Can you work these out from the model? Positions are in its coordinate system, mm. Face numbers are marked on the shaded views. Coordinates: 2 decimals unless noted, no trailing zeros. Loops run counter-clockwise (first coordinate to the right, second up) from the corner with the lowest first, then second, coordinate; pieces in that order, holes last.
```python
from build123d import *

# Parameters (mm, degrees)
F1_DEPTH = 1
F3_DEPTH = 1.4
F4_W     = 2
F4_H     = 10
F4_W_2   = 15
F4_H_2   = 2
F5_DEPTH = 0.6
F6_W     = 1
F6_H     = 119
F7_DEPTH = 0.4


with BuildPart() as f1:
    # F0 (on Top) → F1 (new body)
    with BuildSketch(Plane.XY):
        Polygon((-25, 88.965908), (-45, 88.965908), (-45, -39.534092), (59.5, -39.534092), (59.5, 88.965908), (0, 88.965908), (0, 106.965908), (-25, 106.965908), align=None)
    extrude(amount=F1_DEPTH)

    # F2 (on face) → F3 (join)
    with BuildSketch(Plane.XY.offset(1)):
        Polygon((-37.25, -30.034092), (-37.25, 88.965908), (-45, 88.965908), (-45, -39.534092), (59.5, -39.534092), (59.5, 88.965908), (51.75, 88.965908), (51.75, -30.034092), align=None)
    extrude(amount=F3_DEPTH)

    # F4 (on face) → F5 (join)
    with BuildSketch(Plane.XY.offset(2.4)):
        with Locations((50.75, 70.738149)):
            Rectangle(F4_W, F4_H)
        with Locations((50.75, -6.520228)):
            Rectangle(F4_W, F4_H)
        with Locations((7.25, -29.034092)):
            Rectangle(F4_W_2, F4_H_2)
        with Locations((-36.250001, -6.520228)):
            Rectangle(F4_W, F4_H)
        with Locations((-36.25, 70.738149)):
            Rectangle(F4_W, F4_H)
    extrude(amount=-F5_DEPTH)

    # F6 (on face) → F7 (join)
    with BuildSketch(Plane.XY.offset(1)):
        with Locations((-34.75, 29.465908)):
            Rectangle(F6_W, F6_H)
        with Locations((-30.75, 29.465908)):
            Rectangle(F6_W, F6_H)
        with Locations((-26.75, 29.465908)):
            Rectangle(F6_W, F6_H)
        with Locations((-22.75, 29.465908)):
            Rectangle(F6_W, F6_H)
        with Locations((-18.75, 29.465908)):
            Rectangle(F6_W, F6_H)
        with Locations((-14.75, 29.465908)):
            Rectangle(F6_W, F6_H)
        with Locations((-10.75, 29.465908)):
            Rectangle(F6_W, F6_H)
        with Locations((-6.75, 29.465908)):
            Rectangle(F6_W, F6_H)
        with Locations((-2.75, 29.465908)):
            Rectangle(F6_W, F6_H)
        with Locations((1.25, 29.465908)):
            Rectangle(F6_W, F6_H)
        with Locations((5.25, 29.465908)):
            Rectangle(F6_W, F6_H)
        with Locations((9.25, 29.465908)):
            Rectangle(F6_W, F6_H)
        with Locations((13.25, 29.465908)):
            Rectangle(F6_W, F6_H)
        with Locations((17.25, 29.465908)):
            Rectangle(F6_W, F6_H)
        with Locations((21.25, 29.465908)):
            Rectangle(F6_W, F6_H)
        with Locations((25.25, 29.465908)):
            Rectangle(F6_W, F6_H)
        with Locations((29.25, 29.465908)):
            Rectangle(F6_W, F6_H)
        with Locations((33.25, 29.465908)):
            Rectangle(F6_W, F6_H)
        with Locations((37.25, 29.465908)):
            Rectangle(F6_W, F6_H)
        with Locations((41.25, 29.465908)):
            Rectangle(F6_W, F6_H)
        with Locations((49.25, 29.465908)):
            Rectangle(F6_W, F6_H)
        with Locations((45.25, 29.465908)):
            Rectangle(F6_W, F6_H)
    extrude(amount=F7_DEPTH)


solid = f1.part
```
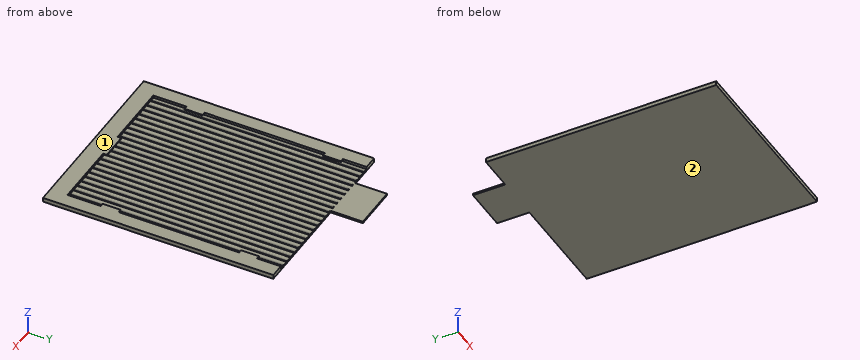
Item 1: We'd pull the mould along Z, two halves only. Please class the marked faces 1 and 2: +Z half, -Z half, draft (parallel to the pull), parting line (faces both ways), or undercut.
Results are:
face 1: +Z half
face 2: -Z half
Item 2: I'm going to push flat-ended pins straight in: P1, Ø0.9, axis at x = 11.5, y = 39, coming from the +Z side; P2, Ø1.6, axis at x = 50.5, y = 27.5, coming from the +Z side; P3, Ø1.2, axis at x = 40.5, z = 1.5, coming from the +Y side. Where does each tip first touch, or does it pass through?
Results are:
P1: stops at z = 1
P2: stops at z = 1.4
P3: stops at y = 88.97
Item 3: Suppose I cut it at A-A, the plane z = 0.6. Please give me the cut outline in (x, y).
Results are:
outline: (-45, -39.53) - (59.5, -39.53) - (59.5, 88.97) - (0, 88.97) - (0, 106.97) - (-25, 106.97) - (-25, 88.97) - (-45, 88.97) - close
Item 4: I need wall thicknesses on line 1 along X through (y, z) = (-9, 1.95); line 2 along X through (y, z) = (60.5, 1.6); line 3 along Y through (x, z) = (-23.5, 1.3). Which ranges of each line are inside material? Lowest first, please.
Results are:
line 1: x = -45 to -35.25, 49.75 to 59.5
line 2: x = -45 to -37.25, 51.75 to 59.5
line 3: y = -39.53 to -30.03
